Could you check a few things on this model? Use its own coordinates, in mm. Face numbers are marked on the shaded views. Coordinates: 2 decimals unless noted, no trailing zeros. Order: outer loops, then holes, each group sorted by start corner. A loop starts at its lowest first (then second) coordinate and runs counter-clockwise, first axis right, second up. Notation, with made-up numbers: (9, 2.5) -> (47, 2.5) arc R27 ccw to (47, 21.5) -> close; hole circle Ø5 at (-11, 86). An arc over 180 degrees is marked (long way). Return JSON: item names as keys, results as strings. Group by question number.
from build123d import *

# Parameters (mm, degrees)
REVOLVE1_ANGLE     = 180
SKETCH2_W          = 10
SKETCH2_H          = 35
CUT_REVOLVE1_ANGLE = 10
SKETCH4_R          = 2.5
CUT_EXTRUDE1_DEPTH = 20
SKETCH5_W          = 10
SKETCH5_H          = 20
REVOLVE2_ANGLE     = 10


with BuildPart() as part:
    # Sketch1 → Revolve1 (revolve)
    with BuildSketch(Plane(origin=(0, 0, 0), x_dir=(1, 0, 0), z_dir=(0, 1, 0))):
        Polygon((-60, 19.117647059), (-60, -80.882352941), (-50, -80.882352941), (-50, -5.882352941), (-55, -5.882352941), (-55, 4.117647059), (-50, 4.117647059), (-50, 19.117647059), align=None)
    revolve(axis=Axis((0, 0, -69.117647059), (0, 0, 1)), revolution_arc=REVOLVE1_ANGLE)

    # Sketch2 → Cut-Revolve1 (revolve, cut)
    with BuildSketch(Plane(origin=(0, 0, 0), x_dir=(1, 0, 0), z_dir=(0, 1, 0))):
        with Locations((-55, -43.382352941)):
            Rectangle(SKETCH2_W, SKETCH2_H)
    revolve(axis=Axis((0, 0, 80.882352941), (0, 0, 1)), revolution_arc=CUT_REVOLVE1_ANGLE, mode=Mode.SUBTRACT)

    # Sketch4 → Cut-Extrude1 (cut)
    with BuildSketch(Plane(origin=(60, 0, 0), x_dir=(0, 0, 1), z_dir=(1, 0, 0))):
        with Locations((35.882352941, 7.5)):
            Circle(SKETCH4_R)
        with Locations((50.882352941, 7.5)):
            Circle(SKETCH4_R)
        with Locations((20.882352941, 7.5)):
            Circle(SKETCH4_R)
    extrude(amount=-CUT_EXTRUDE1_DEPTH, mode=Mode.SUBTRACT)

    # Sketch5 → Revolve2 (revolve)
    with BuildSketch(Plane(origin=(0, 0, 0), x_dir=(1, 0, 0), z_dir=(0, 1, 0))):
        with Locations((-55, -70.882352941)):
            Rectangle(SKETCH5_W, SKETCH5_H)
        with Locations((-55, -15.882352941)):
            Rectangle(SKETCH5_W, SKETCH5_H)
    revolve(axis=Axis((0, 0, 85.860952493), (0, 0, -1)), revolution_arc=REVOLVE2_ANGLE)


solid = part.part
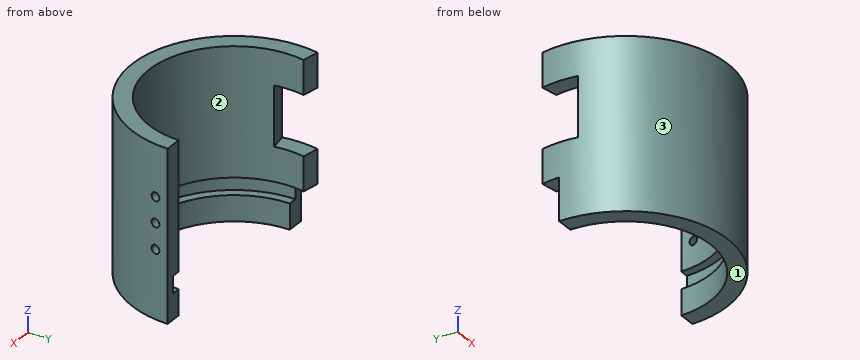
Q1. I need wall thicknesses on line 1 along Z through (x, y) = (53.25, -7.5); line 2 along X through (y, z) = (-0.5, -2); line 3 along Z through (x, y) = (54, -7). Which ranges of each line are inside material? Lowest first, please. Write a range as from..to.
Q2. I'm going to push flat-ended pins straight in: pin 1 Ø6.5 at (y, z) = (-7.5, 20.88) entering from -X; pin 2 Ø8 at (x, z) = (13, 58.5) entering from -Y; pin 3 Ø12 at (y, z) = (-31, -5) entering from +X. Where does each tip first touch, or does it pass through?
Q3. I want a section at B-B on y = -2.5. Please give me the cut outline in (x, z).
Q4. I want a section at A-A on y = -40.5. Please give me the cut outline in (x, z).
Q5. I want a section at C-C on x = 0. Please give me the cut outline in (y, z).
Q6. I want a section at D-D on z = -9.5. Please give me the cut outline in (x, y), and give its area (3 significant figures).
Q7. We'd pull the mould along X, two halves only. Please class the marked faces 1, 2 and 3: pulls with the +X half, pulls with the -X half, needs draft (parallel to the pull), parting line crosses it, or undercut.
Response values:
{
 "1": {"line 1": "z = -19.12..-4.12, 5.88..18.38, 23.38..33.38, 38.38..48.38, 53.38..80.88", "line 2": "x = -60..-55, 55..60", "line 3": "z = -19.12..-4.12, 5.88..18.43, 23.33..33.43, 38.33..48.43, 53.33..80.88"},
 "2": {"pin 1": "stops at x = -59.85", "pin 2": "stops at y = -59.32", "pin 3": "stops at x = 54.54"},
 "3": {"outline": "(-59.95, -19.12) -> (-49.94, -19.12) -> (-49.94, -4.12) -> (-54.94, -4.12) -> (-54.94, 5.88) -> (-49.94, 5.88) -> (-49.94, 25.88) -> (-59.95, 25.88) -> close; (-59.95, 60.88) -> (-49.94, 60.88) -> (-49.94, 80.88) -> (-59.95, 80.88) -> close; (49.94, -19.12) -> (59.95, -19.12) -> (59.95, 80.88) -> (49.94, 80.88) -> (49.94, 5.88) -> (54.94, 5.88) -> (54.94, -4.12) -> (49.94, -4.12) -> close"},
 "4": {"outline": "(-44.27, -19.12) -> (-29.32, -19.12) -> (-29.32, -4.12) -> (-37.21, -4.12) -> (-37.21, 5.88) -> (-29.32, 5.88) -> (-29.32, 80.88) -> (-44.27, 80.88) -> close; (29.32, -19.12) -> (44.27, -19.12) -> (44.27, 80.88) -> (29.32, 80.88) -> (29.32, 5.88) -> (37.21, 5.88) -> (37.21, -4.12) -> (29.32, -4.12) -> close"},
 "5": {"outline": "(-60, -19.12) -> (-50, -19.12) -> (-50, -4.12) -> (-55, -4.12) -> (-55, 5.88) -> (-50, 5.88) -> (-50, 80.88) -> (-60, 80.88) -> close"},
 "6": {"outline": "(-60, 0) arc R60 ccw to (60, 0) -> (50, 0) arc R50 cw to (-50, 0) -> close", "area": "1,730 mm²"},
 "7": {"face 1": "needs draft", "face 2": "undercut", "face 3": "parting line crosses it"}
}
